The drawing under review shows one solid part. Ordinate dimensions are in mm from its lowest x, y, z. A direction names the side the tool comes from. Coordinates: 2 decimals unless noted, no trailing zeros. Write each loop counter-clockwise with the first axis right and the second up, starting at its lowest first coordinate (ties: lowest second). Pieces come first, ordered by that corner, then holes.
1) To check wall thickness, follow line 1 along Z through (x, y) = (8, 10.55); line 2 along Z through (x, y) = (9, 15.25); line 3 along Z through (x, y) = (10, 9.25). State the ranges of each line that lie inside material, in increasing order.
2) We need section A-A on x = 8. Write out the cut boundary in (y, z).
3) We need section D-D on x = 1.5. Write out the cut boundary in (y, z).
4) We need section B-B on z = 23.5. Write out the cut boundary in (x, y), then the cut area to 3 significant figures.
5) For the marked faces 1, 2 and 3, list the 3-axis set-ups (+Z, -Z, +X, -X, +Y, -Y) from which the entire face can be reached by the end or side of a thin tool; tool diameter is ignored.
6) Insertion check: P1, Ø6, axis at y = 13.5, z = 5, coming from the -X side; P2, Ø6, axis at y = 7.5, z = 24.5, coming from the -X side. Each pin has a flat end and moves straight along its axis. Give the tip position at first contact, or say it passes through.
7) We need section C-C on y = 12.5. Write out the cut boundary in (x, z), then the cut area to 3 significant figures.
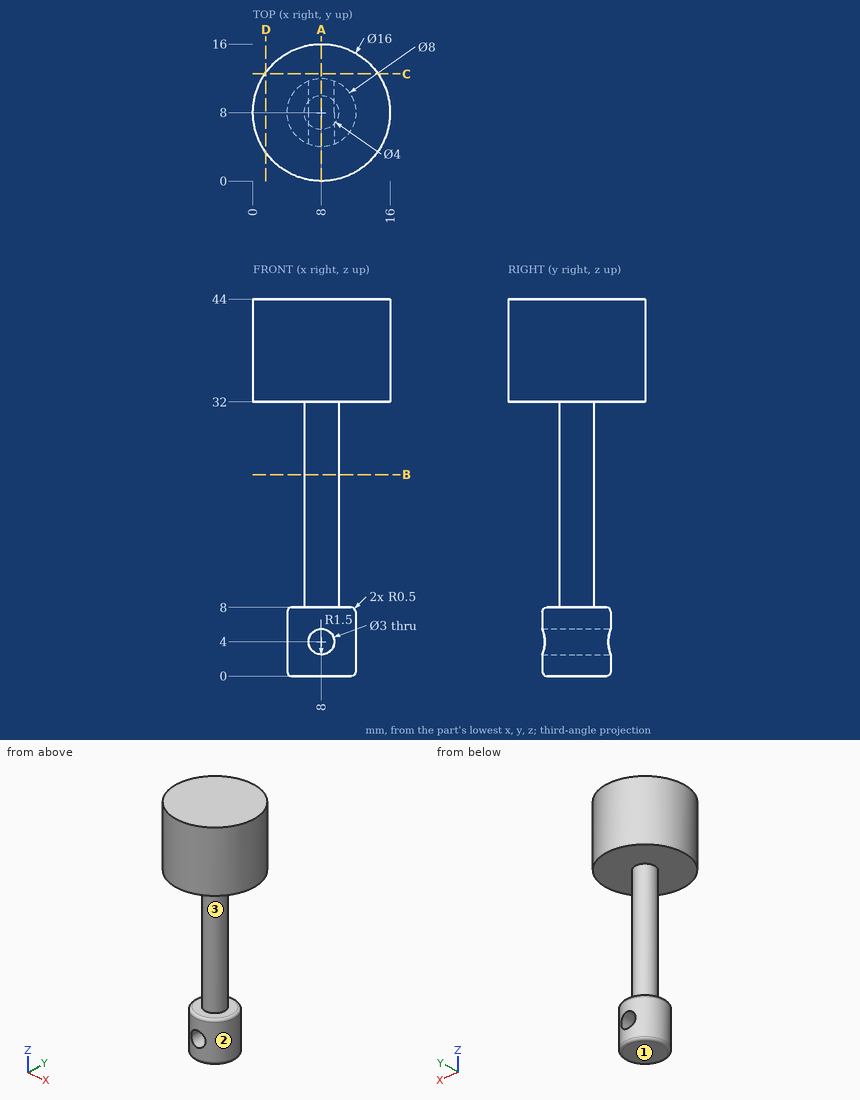
Result:
1. line 1: z = 0 to 2.5, 5.5 to 8, 32 to 44
1. line 2: z = 32 to 44
1. line 3: z = 0 to 8, 32 to 44
2. outline: (0, 32) - (6, 32) - (6, 8) - (4.5, 8) arc R0.5 ccw to (4, 7.5) - (4, 5.5) - (12, 5.5) - (12, 7.5) arc R0.5 ccw to (11.5, 8) - (10, 8) - (10, 32) - (16, 32) - (16, 44) - (0, 44) - close; (4, 0.5) arc R0.5 ccw to (4.5, 0) - (11.5, 0) arc R0.5 ccw to (12, 0.5) - (12, 2.5) - (4, 2.5) - close
3. outline: (3.34, 32) - (12.66, 32) - (12.66, 44) - (3.34, 44) - close
4. outline: circle Ø4 at (8, 8)
4. area: 12.6 mm2
5. face 1: -Z, +X, -X, +Y, -Y
5. face 2: -Z
5. face 3: none
6. P1: stops at x = 4.88
6. P2: stops at x = 6
7. outline: (1.39, 32) - (14.61, 32) - (14.61, 44) - (1.39, 44) - close
7. area: 159 mm2
